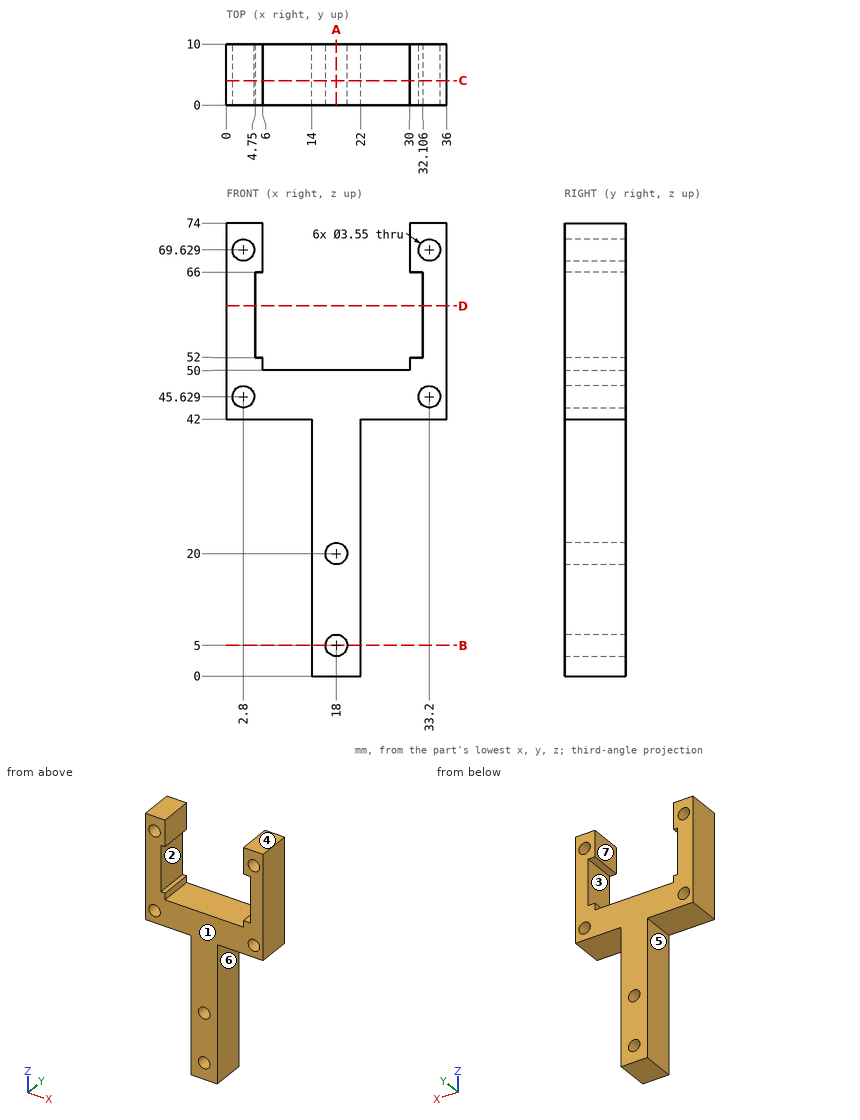
Here's the drawing with two shaded views (mm, measured from the low corner). I have some questions. A direction names the side the tool comes from. Coordinates: 2 decimals unless noted, no trailing zeros. Loops run counter-clockwise (first coordinate to the right, second up) from the corner with the lowest first, then second, coordinate; pieces in that order, holes last. Notation, with made-up numbers: (-30, 80) -> (-24, 80) arc R35 cw to (-24, 119) -> close; hole circle Ø3 at (83, -13). An arc over 180 degrees is marked (long way). Answer as a JSON object with one key per item and string values.
1) Imagine slicing it at D-D (z = 60.5). Please give me the cut outline in (x, y).
Results:
{"outline": "(0, 0) -> (4.75, 0) -> (4.75, 10) -> (0, 10) -> close; (32.11, 0) -> (36, 0) -> (36, 10) -> (32.11, 10) -> close"}
2) Thinking about a two-plate mould opening in Z: for the marked faces 1, 2, 3 and 4, which applies, pulls with the +Z half, pulls with the -Z half, needs draft (parallel to the pull), parting line crosses it, or undercut?
Results:
{"face 1": "needs draft", "face 2": "undercut", "face 3": "undercut", "face 4": "pulls with the +Z half"}
3) For the marked faces 5, 6 and 7, which set-ups out of +Z, -Z, +X, -X, +Y, -Y let a thin tool reach every point of the face, with its end or its side?
Results:
{"face 5": "-Z, -X, +Y, -Y", "face 6": "-Z, +X, +Y, -Y", "face 7": "+Z, +Y, -Y"}
4) Imagine slicing it at B-B (z = 5). Please give me the cut outline in (x, y) (1 decimal), then the cut area to 3 significant figures.
Results:
{"outline": "(14, 0) -> (16.2, 0) -> (16.2, 10) -> (14, 10) -> close; (19.8, 0) -> (22, 0) -> (22, 10) -> (19.8, 10) -> close", "area": "44.5 mm^2"}
5) Imagine slicing it at C-C (y = 4). Count the separate pieces of the cut face and the enclosed holes in it.
Results:
{"separate pieces": "1", "enclosed holes": "6"}
6) Imagine slicing it at A-A (x = 18). Please give me the cut outline in (y, z) (1 decimal), then the cut area to 3 significant figures.
Results:
{"outline": "(0, 0) -> (10, 0) -> (10, 3.2) -> (0, 3.2) -> close; (0, 6.8) -> (10, 6.8) -> (10, 18.2) -> (0, 18.2) -> close; (0, 21.8) -> (10, 21.8) -> (10, 50) -> (0, 50) -> close", "area": "429 mm^2"}
7) If I drill on line 1 (Z direction, x = 33.2, y = 2.5); line 2 (Z direction, x = 19, y = 9.25) (1 decimal); line 3 (X direction, y = 6, z = 46.5), over which ranges is the centre line in solid material (lowest first)?
Results:
{"line 1": "z = 42 to 43.85, 47.4 to 67.85, 71.4 to 74", "line 2": "z = 0 to 3.5, 6.5 to 18.5, 21.5 to 50", "line 3": "x = 0 to 1.25, 4.35 to 31.65, 34.75 to 36"}
8) For P1, Ø3, axis at y = 3, z = 12.5, coming from the -X side; P2, Ø2, axis at x = 20, y = 3.5, coming from the +Z side; P3, Ø1.5, axis at x = 11.5, z = 19, coming from the +Y side; P4, Ø1.4, axis at x = 5.5, y = 4.5, coming from the -Z side, each with a flat end and sliding along its axis, tell me the tip position at first contact or that it passes through.
Results:
{"P1": "stops at x = 14", "P2": "stops at z = 50", "P3": "passes through", "P4": "stops at z = 42"}
